Geometry check sheet. Reference: the model listing, model coordinates, mm. Coordinates: 2 decimals unless noted, no trailing zeros. Write each loop counter-clockwise with the first axis right and the second up, starting at its lowest first coordinate (ties: lowest second). Pieces come first, ordered by that corner, then holes. Notation, with made-up numbers: (38, 43) -> (51, 43) arc R21 cw to (51, 68) -> close; hole circle Ø2 at (18, 45). An arc over 180 degrees is marked (long way). Answer as CSV lines item,"result".
```python
from build123d import *

# Parameters (mm, degrees)
F1_DEPTH = 1.5875
F2_D     = 3
F2_DEPTH = 5
F3_D     = 3
F3_DEPTH = 5
F5_DEPTH = 25
F7_DEPTH = 25
F9_DEPTH = 25


with BuildPart() as f1:
    # F0 (on Top) → F1 (new body)
    with BuildSketch(Plane.XY):
        with BuildLine():
            Line((10.5, 13.5), (-13.5, 13.5))
            Line((-13.5, 13.5), (-27.4, 13.5))
            ThreePointArc((-27.4, 13.5), (-29.52132, 12.62132), (-30.4, 10.5))
            Line((-30.4, 10.5), (-30.4, -10.5))
            ThreePointArc((-30.4, -10.5), (-29.52132, -12.62132), (-27.4, -13.5))
            Line((-27.4, -13.5), (-13.5, -13.5))
            Line((-13.5, -13.5), (10.5, -13.5))
            ThreePointArc((10.5, -13.5), (12.480835, -12.753063), (13.475297, -10.884196))
            ThreePointArc((13.475297, -10.884196), (14.001534, -9.895254), (15.049725, -9.5))
            Line((15.049725, -9.5), (34.5, -9.5))
            ThreePointArc((34.5, -9.5), (36.62132, -8.62132), (37.5, -6.5))
            Line((37.5, -6.5), (37.5, 6.5))
            ThreePointArc((37.5, 6.5), (36.62132, 8.62132), (34.5, 9.5))
            Line((34.5, 9.5), (15.049725, 9.5))
            ThreePointArc((15.049725, 9.5), (14.001534, 9.895254), (13.475297, 10.884196))
            ThreePointArc((13.475297, 10.884196), (12.480835, 12.753063), (10.5, 13.5))
        make_face()
    extrude(amount=-F1_DEPTH)

    # F2
    with Locations(Plane.XY):
        with Locations((-10, 10), (10, 10), (10, -10), (-10, -10)):
            Hole(F2_D / 2, depth=F2_DEPTH)

    # F3
    with Locations(Plane.XY):
        with Locations((-28.64, 8.5), (-16.04, -8.5)):
            Hole(F3_D / 2, depth=F3_DEPTH)

    # F4 (on face) → F5 (cut)
    with BuildSketch(Plane.XY):
        with BuildLine():
            Line((5.695932, 10), (-5.695932, 10))
            ThreePointArc((-5.695932, 10), (-6.603693, 9.714854), (-7.185351, 8.961853))
            ThreePointArc((-7.185351, 8.961853), (-7.87868, 7.87868), (-8.961853, 7.185351))
            ThreePointArc((-8.961853, 7.185351), (-9.714854, 6.603693), (-10, 5.695932))
            Line((-10, 5.695932), (-10, -5.695932))
            ThreePointArc((-10, -5.695932), (-9.714854, -6.603693), (-8.961853, -7.185351))
            ThreePointArc((-8.961853, -7.185351), (-7.87868, -7.87868), (-7.185351, -8.961853))
            ThreePointArc((-7.185351, -8.961853), (-6.603693, -9.714854), (-5.695932, -10))
            Line((-5.695932, -10), (5.695932, -10))
            ThreePointArc((5.695932, -10), (6.603693, -9.714854), (7.185351, -8.961853))
            ThreePointArc((7.185351, -8.961853), (7.87868, -7.87868), (8.961853, -7.185351))
            ThreePointArc((8.961853, -7.185351), (9.714854, -6.603693), (10, -5.695932))
            Line((10, -5.695932), (10, 5.695932))
            ThreePointArc((10, 5.695932), (9.714854, 6.603693), (8.961853, 7.185351))
            ThreePointArc((8.961853, 7.185351), (7.87868, 7.87868), (7.185351, 8.961853))
            ThreePointArc((7.185351, 8.961853), (6.603693, 9.714854), (5.695932, 10))
        make_face()
    extrude(amount=-F5_DEPTH, mode=Mode.SUBTRACT)

    # F6 (on face) → F7 (cut)
    with BuildSketch(Plane.XY):
        with BuildLine():
            Line((-15, 12), (-24.658826, 12))
            ThreePointArc((-24.658826, 12), (-26.467781, 10.853044), (-26.201944, 8.727684))
            Line((-26.201944, 8.727684), (-16.543118, -2.986947))
            ThreePointArc((-16.543118, -2.986947), (-14.324069, -3.596948), (-13, -1.714631))
            Line((-13, -1.714631), (-13, 10))
            ThreePointArc((-13, 10), (-13.585786, 11.414214), (-15, 12))
        make_face()
        with BuildLine():
            Line((-19.456882, -4.168822), (-25.356882, 2.986947))
            ThreePointArc((-25.356882, 2.986947), (-27.575931, 3.596948), (-28.9, 1.714631))
            Line((-28.9, 1.714631), (-28.9, -10))
            ThreePointArc((-28.9, -10), (-28.314214, -11.414214), (-26.9, -12))
            Line((-26.9, -12), (-21, -12))
            ThreePointArc((-21, -12), (-19.585786, -11.414214), (-19, -10))
            Line((-19, -10), (-19, -5.441137))
            ThreePointArc((-19, -5.441137), (-19.117683, -4.765207), (-19.456882, -4.168822))
        make_face()
    extrude(amount=-F7_DEPTH, mode=Mode.SUBTRACT)

    # F8 (on face) → F9 (cut)
    with BuildSketch(Plane.XY):
        with BuildLine():
            ThreePointArc((26.728809, 3.554025), (27.436578, 5.338867), (25.907406, 6.5))
            Line((25.907406, 6.5), (14.5875, 6.5))
            ThreePointArc((14.5875, 6.5), (13.464968, 6.035032), (13, 4.9125))
            Line((13, 4.9125), (13, -1.932094))
            ThreePointArc((13, -1.932094), (13.807699, -3.314869), (15.408903, -3.290569))
            Line((15.408903, -3.290569), (26.728809, 3.554025))
        make_face()
        with BuildLine():
            Line((21.592594, -6.5), (32.9125, -6.5))
            ThreePointArc((32.9125, -6.5), (34.035032, -6.035032), (34.5, -4.9125))
            Line((34.5, -4.9125), (34.5, 1.932094))
            ThreePointArc((34.5, 1.932094), (33.692301, 3.314869), (32.091097, 3.290569))
            Line((32.091097, 3.290569), (20.771191, -3.554025))
            ThreePointArc((20.771191, -3.554025), (20.063422, -5.338867), (21.592594, -6.5))
        make_face()
    extrude(amount=-F9_DEPTH, mode=Mode.SUBTRACT)


solid = f1.part
```
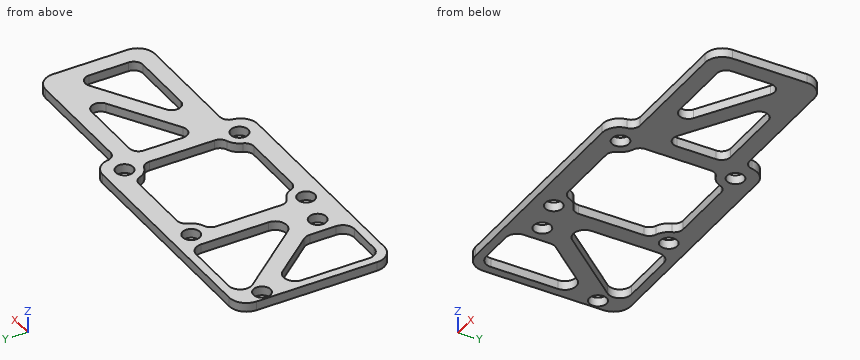
Item 1: Depth check by flat-ended pin: pin 1 Ø1 at (x, y) = (5.5, -10.5) entering from +Z; pin 2 Ø2.5 at (x, y) = (-10, -10) entering from +Z; pin 3 Ø0.5 at (x, z) = (20.5, -0.5) entering from -Y. Enter the tip coordinate at first touch or a pass-through.
Responses:
pin 1,"stops at z = 0"
pin 2,"passes through"
pin 3,"stops at y = -9.5"
Item 2: Cross-section at C-C, the plane x = 29.5. Record the cut outline in (y, z), plus the area to 3 significant figures.
Responses:
outline,"(-9.5, -1.59) -> (-6.5, -1.59) -> (-6.5, 0) -> (-9.5, 0) -> close; (1.72, -1.59) -> (9.5, -1.59) -> (9.5, 0) -> (1.72, 0) -> close"
area,"17.1 mm2"
Item 3: Cross-section at B-B, the plane z = -1.05. Count the separate pieces of the cut face and the enclosed holes in it, plus the area to 3 significant figures.
Responses:
separate pieces,"1"
enclosed holes,"11"
area,"760 mm2"
Item 4: Thickness scan on probe 1 along X at (y, z) = (-8.75, -0.7); probe 2 along X at (y, z) = (10.5, -0.2); probe 3 along Y at (x, z) = (27, -0.25). Record the ranges inside material, lowest first.
Responses:
probe 1,"x = -30.4 to -28.9, -19 to -17.52, -14.56 to -10.83, -9.17 to -7.27, 7.27 to 9.17, 10.83 to 36.48"
probe 2,"x = -30.4 to -26.6, -13.06 to -11.41, -8.59 to 8.59, 11.41 to 13.57"
probe 3,"y = -9.5 to -6.5, 0.21 to 3.76, 6.06 to 9.5"
Item 5: Cross-section at A-A, the plane x = 0.5. Record the cut outline in (y, z).
Responses:
outline,"(-13.5, -1.59) -> (-10, -1.59) -> (-10, 0) -> (-13.5, 0) -> close; (10, -1.59) -> (13.5, -1.59) -> (13.5, 0) -> (10, 0) -> close"
